Input: part model. Units: mm. Frame: model coordinates. Round coordinates to 2 decimals unless told otherwise and drop trailing zeros. Order: outer loops, then holes, each group sorted by start corner. A loop starts at its lowest first (then second) coordinate and runs counter-clockwise, first axis right, second up. Notation, with made-up numbers: (57.5, -2.75) -> (65.5, -2.75) arc R17 cw to (65.5, 22.25) -> close; hole circle Ø2 at (39, 47). An arc over 180 degrees is marked (long way). Use a Markdown table: item, result.
from build123d import *

# Parameters (mm, degrees)
BOSS_EXTRUDE1_DEPTH = 20
SKETCH3_R           = 10.5
CUT_EXTRUDE1_DEPTH  = 42.851672607
SKETCH4_R           = 1.1
CUT_EXTRUDE2_DEPTH  = 2.5
FILLET1_R           = 0.5


with BuildPart() as part:
    # Sketch1 → Boss-Extrude1 (new body)
    with BuildSketch(Plane.XY):
        with BuildLine():
            Line((10, 1.25), (30, 1.25))
            Line((30, 1.25), (30, -1.25))
            Line((30, -1.25), (-30, -1.25))
            Line((-30, -1.25), (-30, 1.25))
            Line((-30, 1.25), (-10, 1.25))
            ThreePointArc((-10, 1.25), (0, 21.25), (10, 1.25))
        make_face()
    extrude(amount=BOSS_EXTRUDE1_DEPTH)

    # Sketch3 → Cut-Extrude1 (cut, through all)
    with BuildSketch(Plane.XY.offset(20)):
        with Locations((0, 8.75)):
            Circle(SKETCH3_R)
    extrude(amount=-CUT_EXTRUDE1_DEPTH, mode=Mode.SUBTRACT)

    # Sketch4 → Cut-Extrude2 (cut)
    with BuildSketch(Plane(origin=(0, 1.25, 0), x_dir=(1, 0, 0), z_dir=(0, 1, 0))):
        with Locations(Location((-20, -10, 0), (0, 0, 270))):
            Circle(SKETCH4_R)
        with Locations(Location((20, -10, 0), (0, 0, 270))):
            Circle(SKETCH4_R)
    extrude(amount=-CUT_EXTRUDE2_DEPTH, mode=Mode.SUBTRACT)

    # Fillet1
    fillet1_edges = [part.edges().sort_by_distance(p)[0] for p in [
        (-3.201562119, -1.25, 10),
        (3.201562119, -1.25, 10),
    ]]
    fillet(fillet1_edges, radius=FILLET1_R)


solid = part.part
1) Pin query (flat end, axial travel): pin 1 Ø2.5 at (x, z) = (20, 10) entering from +Y; pin 2 Ø6 at (x, z) = (12.5, 9) entering from +Y; pin 3 Ø12 at (y, z) = (11, 9) entering from +X. Return the tip coordinate at first contact, or that it passes through.
Results found:
| item | result |
|---|---|
| pin 1 | stops at y = 1.25 |
| pin 2 | stops at y = 16.87 |
| pin 3 | stops at x = 12.5 |
2) Line query: L1, parallel to X at y = -0.55, z = 10; L2, parallel to X at y = 9.25, z = 4.75; L3, parallel to Y at x = 0, z = 11.5. Output: solid intervals per line, ascending. Write a range as [from, to].
Results found:
| item | result |
|---|---|
| L1 | x = [-30, -21.1], [-18.9, -5.09], [5.09, 18.9], [21.1, 30] |
| L2 | x = [-12.49, -10.49], [10.49, 12.49] |
| L3 | y = [19.25, 21.25] |
3) Cut plane A-A on x = -20. Return loops of the section in (y, z), and give its area (3 significant figures).
Results found:
| item | result |
|---|---|
| outline | (-1.25, 0) -> (1.25, 0) -> (1.25, 8.9) -> (-1.25, 8.9) -> close; (-1.25, 11.1) -> (1.25, 11.1) -> (1.25, 20) -> (-1.25, 20) -> close |
| area | 44.5 mm² |
4) Cut plane B-B on z = 10. Return loops of the section in (x, y), and give its area (3 significant figures).
Results found:
| item | result |
|---|---|
| outline | (-30, -1.25) -> (-21.1, -1.25) -> (-21.1, 1.25) -> (-30, 1.25) -> close; (-18.9, -1.25) -> (-5.55, -1.25) arc R0.5 ccw to (-5.29, -0.32) arc R10.5 cw (long way) to (5.29, -0.32) arc R0.5 ccw to (5.55, -1.25) -> (18.9, -1.25) -> (18.9, 1.25) -> (10, 1.25) arc R12.5 ccw (long way) to (-10, 1.25) -> (-18.9, 1.25) -> close; (21.1, -1.25) -> (30, -1.25) -> (30, 1.25) -> (21.1, 1.25) -> close |
| area | 214 mm² |
5) Cut plane D-D on x = 0. Return loops of the section in (y, z), and give its area (3 significant figures).
Results found:
| item | result |
|---|---|
| outline | (19.25, 0) -> (21.25, 0) -> (21.25, 20) -> (19.25, 20) -> close |
| area | 40.0 mm² |
6) Cut plane C-C on y = 14.75. Return loops of the section in (x, z), and give its area (3 significant figures).
Results found:
| item | result |
|---|---|
| outline | (-10.97, 0) -> (-8.62, 0) -> (-8.62, 20) -> (-10.97, 20) -> close; (8.62, 0) -> (10.97, 0) -> (10.97, 20) -> (8.62, 20) -> close |
| area | 94.0 mm² |
7) Pull-direction query (Y, two-part tool) for faces 1 (the flat face through (-18, -1.25, 10)), 2 (the flat face through (7, 0, 0)), 3 (the cylindrical face through (0.384, 19.243, 10.14)); classes: +Y half, -Y half, draft (parallel to the pull), parting line (faces both ways), or undercut.
Results found:
| item | result |
|---|---|
| face 1 | -Y half |
| face 2 | draft |
| face 3 | undercut |
